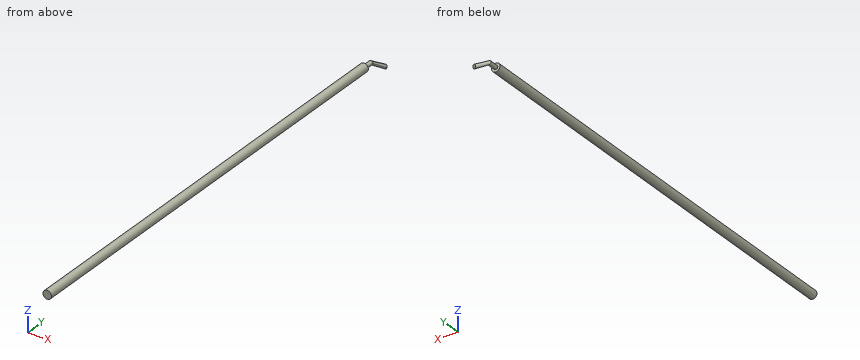
Autodesk Inventor part; units mm, degrees
ref_plane "YZ Plane" through (0, 0, 0) normal (1, 0, 0) x (0, 1, 0)
ref_plane "XZ Plane" through (0, 0, 0) normal (0, 1, 0) x (-1, 0, 0)
ref_plane "XY Plane" through (0, 0, 0) normal (0, 0, 1) x (1, 0, 0)
ref_plane "Work Plane2" through (3.5859, 0, -0.978) normal (0, -1, 0) x (1, 0, 0)
sketch "Sketch2" plane through (3.5859, 0, -0.978) normal (0, -1, 0) x (1, 0, 0)
  circle A0 centre (0, 0) radius 0.675
  point P0 (-3.5859, 0.978)
  dimension "d3" = 1.35
extrude "Extrusion2" add sketch "Sketch2" along normal blind 71.25
ref_plane "Work Plane1" through (3.5859, 3, -0.978) normal (0, 1, 0) x (1, 0, 0)
sketch "Sketch3" plane through (3.5859, 0, -0.978) normal (0, 1, 0) x (1, 0, 0)
  circle A0 centre (0, 0) radius 0.315
  point P0 (-3.5859, -0.978)
  dimension "d7" = 0.63
extrude "Extrusion3" add sketch "Sketch3" along normal blind 1.5
ref_plane "Work Plane3" through (5.9115, 2.4915, -1.92) normal (0.4330127, 0.8660254, -0.25) x (0.5, 0, 0.8660254)
sketch "Sketch5" plane through (5.9115, 2.4915, -1.92) normal (0.4330127, 0.8660254, -0.25) x (0.5, 0, 0.8660254)
  circle A0 centre (-0.4635, -1.064) radius 0.315
  point P0 (-1.293, -4.0192)
  dimension "d11" = 0.63
loft "Loft1" add profiles "Sketch5" section 1 edges at (3.2709, 1.5, -0.978)
properties part number "redWire"
Source: CAD feature listing. Evaluate the final solid. Frame: model axes, mm. Round coordinates to 2 decimals unless told otherwise and drop trailing zeros. Order: outer loops, then holes, each group sorted by start corner. A loop starts at its lowest first (then second) coordinate and runs counter-clockwise, first axis right, second up. Notation, with made-up numbers: (50, -32) -> (55, -32) arc R34 ccw to (55, -1) -> close; hole circle Ø4 at (-7.75, 64). An arc over 180 degrees is marked (long way). Answer as CSV lines item,"result".
Item 1: Section A-A, the plane y = -29. Return loops of the section in (x, z) (3 decimals), plus the area to 3 significant figures.
A:
outline,"circle Ø1.35 at (3.586, -0.978)"
area,"1.43 mm²"
Item 2: Pin query (flat end, axial travel): pin 1 Ø1 at (y, z) = (-58, -1.5) entering from +X. Return the tip coordinate at first contact, or that it passes through.
A:
pin 1,"x = 4.26"
Item 3: Line query: L1, parallel to Z at x = 3.7, y = -10; L2, parallel to Y at x = 3.45, z = -0.6; L3, parallel to Y at x = 4.95, z = -1.75. Output: solid intervals per line, ascending.
A:
L1,"-1.64 to -0.31"
L2,"-71.25 to 0"
L3,"2.65 to 3.02"
